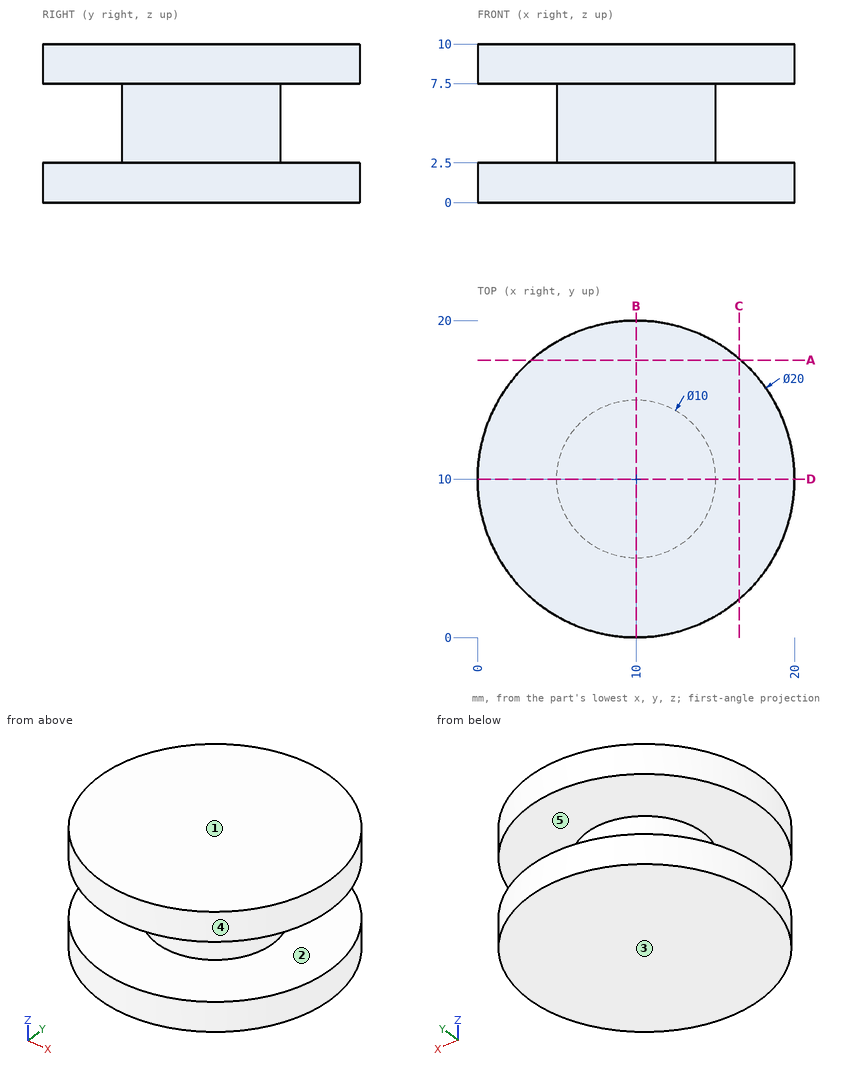
Input: dimensioned drawing with shaded views. Units: mm. Origin: part minimum x, y, z. A direction names the side the tool comes from. Give positions to 0.01 mm unless a question says otherwise; leave off trailing zeros. Loops run counter-clockwise (first coordinate to the right, second up) from the corner with the lowest first, then second, coordinate; pieces in that order, holes last. Notation, with made-up numbers: M -37,63 L -7,63 A22 ccw -7,72 Z; hole C 10.25,84 d9. An arc over 180 degrees is marked long. Put each result on its own line as item: value.
1) First-contact query: P1, Ø5, axis at y = 7, z = 3.5, coming from the -X side; P2, Ø2, axis at x = 3, z = 3, coming from the +Y side. Flat tips, straight axial feed; report the tip coordinate or a pass-through.
Computed values:
P1: stops at x = 0.03
P2: stops at y = 17.9
2) Reachability of the marked faces 4 and 5 from +Z, -Z, +X, -X, +Y, -Y: full face, straight path, thin tool, end or side. Return the list, or none.
Computed values:
face 4: +Z, -Z
face 5: none
3) Cut plane A-A, the plane y = 17.5. Return the cut outline in (x, z).
Computed values:
outline: M 3.39,0 L 16.61,0 L 16.61,2.5 L 3.39,2.5 Z; M 3.39,7.5 L 16.61,7.5 L 16.61,10 L 3.39,10 Z
4) Cut plane B-B, the plane x = 10. Return the cut outline in (y, z).
Computed values:
outline: M 0,0 L 20,0 L 20,2.5 L 15,2.5 L 15,7.5 L 20,7.5 L 20,10 L 0,10 L 0,7.5 L 5,7.5 L 5,2.5 L 0,2.5 Z
5) Cut plane C-C, the plane x = 16.5. Return the cut outline in (y, z), plus the area to 3 significant figures.
Computed values:
outline: M 2.4,0 L 17.6,0 L 17.6,2.5 L 2.4,2.5 Z; M 2.4,7.5 L 17.6,7.5 L 17.6,10 L 2.4,10 Z
area: 76.0 mm^2
6) Material intervals for L1, parallel to Z at x = 7.5, y = 2.75; L2, parallel to Y at x = 2.5, z = 0.5; L3, parallel to Y at x = 10.75, z = 0.75, sorted ascending. Write a range as from..to.
Computed values:
L1: z = 0..2.5, 7.5..10
L2: y = 3.39..16.61
L3: y = 0.03..19.97
7) Mould query, pull axis Z, two halves, no side actions, for the marked faces 1, 2 and 3. Classes: released by +Z, released by -Z, zero draft, split by the parting line, or undercut.
Computed values:
face 1: released by +Z
face 2: undercut
face 3: released by -Z
